Work out the finished part from the listing and answer in its coordinate system (mm). Face numbers are marked on the shaded views. A direction names the side the tool comes from. Round coordinates to 2 decimals unless told otherwise and drop trailing zeros. Loops run counter-clockwise (first coordinate to the right, second up) from the corner with the lowest first, then second, coordinate; pieces in that order, holes last. Notation, with made-up numbers: (31, -4) - (48, -4) arc R18 cw to (48, 19) - close; hole circle Ø10 at (-20.75, 17.25). An arc over 180 degrees is marked (long way). Return JSON: item names as keys, results as strings.
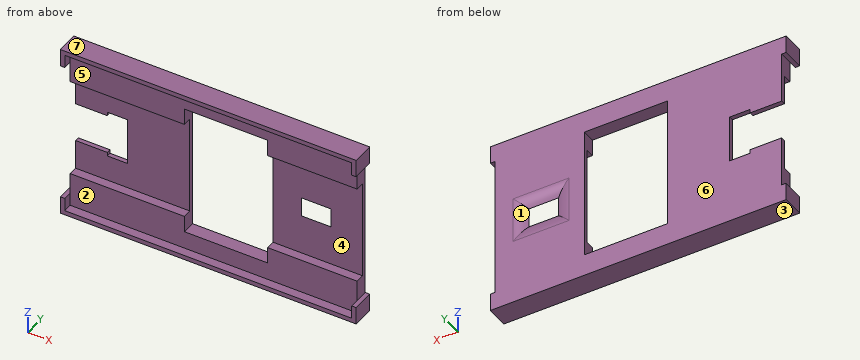
from build123d import *

# Parameters (mm, degrees)
BOSS_EXTRUDE1_DEPTH     = 3
SKETCH2_W               = 6.7
SKETCH2_H               = 4.4
SKETCH2_W_2             = 18.84
SKETCH2_H_2             = 30
CUT_EXTRUDE1_DEPTH      = 77.380625816
CUT_EXTRUDE2_DEPTH      = 61.059054272
CUT_EXTRUDE2_DEPTH_BACK = 61.059054272
SKETCH5_W               = 22.5
SKETCH5_H               = 2
FILLET3_R               = 5
BOSS_EXTRUDE2_DEPTH     = 5


with BuildPart() as part:
    # Sketch1 → Boss-Extrude1 (new body)
    with BuildSketch(Plane(origin=(0, 0, 0), x_dir=(1, 0, 0), z_dir=(0, 1, 0))):
        Polygon((65, -38), (65, -40), (63, -40), (2, -40), (0, -40), (0, -38), (0, -2), (0, 0), (2, 0), (63, 0), (65, 0), (65, -2), align=None)
    extrude(amount=BOSS_EXTRUDE1_DEPTH)

    # Sketch2 → Cut-Extrude1 (cut, through all)
    with BuildSketch(Plane(origin=(0, 3, 0), x_dir=(1, 0, 0), z_dir=(0, 1, 0))):
        with Locations((54.5, -20)):
            Rectangle(SKETCH2_W, SKETCH2_H)
        Polygon((11.78, -25.35), (7.19, -25.35), (7.19, -24.5), (-0.16, -24.5), (-0.16, -15.5), (7.19, -15.5), (7.19, -14.65), (11.78, -14.65), align=None)
        with Locations((35.28, -20)):
            Rectangle(SKETCH2_W_2, SKETCH2_H_2)
    extrude(amount=-CUT_EXTRUDE1_DEPTH, mode=Mode.SUBTRACT)

    # Sketch5 → Cut-Extrude2 (cut, two sides: drawn at the far end of the back side and taken through both)
    with BuildSketch(Plane.ZY.offset(-44.7).offset(-CUT_EXTRUDE2_DEPTH_BACK)):
        with Locations((20, 1)):
            Rectangle(SKETCH5_W, SKETCH5_H)
    extrude(amount=CUT_EXTRUDE2_DEPTH + CUT_EXTRUDE2_DEPTH_BACK, mode=Mode.SUBTRACT)

    # Fillet3
    # the kernel refuses this fillet: 5 mm, written as the material it takes off along each edge
    with BuildSketch(Plane(origin=(57.85, 3, 22.2), x_dir=(0, 0, 1), z_dir=(-1, 0, 0)), Plane(origin=(51.15, 3, 17.8), x_dir=(0, 0, -1), z_dir=(1, 0, 0))) as fillet3_piece_1:
        with BuildLine():
            CenterArc((3, -5), FILLET3_R, 90, 36.869897646)
            Line((0, -1), (-0.06, -0.92))
            ThreePointArc((-0.06, -0.92), (-0.1, -0.5), (-0.1, 0))
            Line((-0.1, 0), (0, 0.1))
            Line((0, 0.1), (3, 0.1))
            Line((3, 0.1), (3, 0))
        make_face()
    extrude(amount=6.7, mode=Mode.SUBTRACT)
    with BuildSketch(Plane(origin=(57.85, 3, 17.8), x_dir=(1, 0, 0), z_dir=(0, 0, 1)), Plane(origin=(51.15, 3, 22.2), x_dir=(-1, 0, 0), z_dir=(0, 0, -1))) as fillet3_piece_2:
        with BuildLine():
            CenterArc((3, -5), FILLET3_R, 90, 36.869897646)
            Line((0, -1), (-0.06, -0.92))
            ThreePointArc((-0.06, -0.92), (-0.1, -0.5), (-0.1, 0))
            Line((-0.1, 0), (0, 0.1))
            Line((0, 0.1), (3, 0.1))
            Line((3, 0.1), (3, 0))
        make_face()
    extrude(amount=4.4, mode=Mode.SUBTRACT)
    with BuildSketch(Plane(origin=(57.85, 3, 17.8), x_dir=(1, 0, 0), z_dir=(0, 0, 1))) as fillet3_piece_3a_section:
        with BuildLine():
            CenterArc((3, -5), FILLET3_R, 90, 36.869897646)
            Line((0, -1), (-0.06, -0.92))
            ThreePointArc((-0.06, -0.92), (-0.1, -0.5), (-0.1, 0))
            Line((-0.1, 0), (0, 0.1))
            Line((0, 0.1), (3, 0.1))
            Line((3, 0.1), (3, 0))
        make_face()
    fillet3_piece_3a = extrude(amount=11.9, mode=Mode.PRIVATE)
    fillet3_piece_3a = split(fillet3_piece_3a, bisect_by=Plane(origin=(58.699672813, 2.773811602, 22.2), z_dir=(0, 0, 1)), keep=Keep.TOP, mode=Mode.PRIVATE)
    with BuildSketch(Plane(origin=(65.35, 3, 22.2), x_dir=(0, 0, 1), z_dir=(-1, 0, 0))) as fillet3_piece_3b_section:
        with BuildLine():
            CenterArc((3, -5), FILLET3_R, 90, 36.869897646)
            Line((0, -1), (-0.06, -0.92))
            ThreePointArc((-0.06, -0.92), (-0.1, -0.5), (-0.1, 0))
            Line((-0.1, 0), (0, 0.1))
            Line((0, 0.1), (3, 0.1))
            Line((3, 0.1), (3, 0))
        make_face()
    fillet3_piece_3b = extrude(amount=14.2, mode=Mode.PRIVATE)
    fillet3_piece_3b = split(fillet3_piece_3b, bisect_by=Plane(origin=(57.85, 2.773811602, 23.049672813), z_dir=(1, 0, 0)), keep=Keep.TOP, mode=Mode.PRIVATE)
    fillet3_piece_3 = fillet3_piece_3a & fillet3_piece_3b
    add(fillet3_piece_3, mode=Mode.SUBTRACT)
    with BuildSketch(Plane(origin=(57.85, 3, 22.2), x_dir=(0, 0, 1), z_dir=(-1, 0, 0))) as fillet3_piece_4a_section:
        with BuildLine():
            CenterArc((3, -5), FILLET3_R, 90, 36.869897646)
            Line((0, -1), (-0.06, -0.92))
            ThreePointArc((-0.06, -0.92), (-0.1, -0.5), (-0.1, 0))
            Line((-0.1, 0), (0, 0.1))
            Line((0, 0.1), (3, 0.1))
            Line((3, 0.1), (3, 0))
        make_face()
    fillet3_piece_4a = extrude(amount=14.2, mode=Mode.PRIVATE)
    fillet3_piece_4a = split(fillet3_piece_4a, bisect_by=Plane(origin=(51.15, 2.773811602, 23.049672813), z_dir=(-1, 0, 0)), keep=Keep.TOP, mode=Mode.PRIVATE)
    with BuildSketch(Plane(origin=(51.15, 3, 29.7), x_dir=(-1, 0, 0), z_dir=(0, 0, -1))) as fillet3_piece_4b_section:
        with BuildLine():
            CenterArc((3, -5), FILLET3_R, 90, 36.869897646)
            Line((0, -1), (-0.06, -0.92))
            ThreePointArc((-0.06, -0.92), (-0.1, -0.5), (-0.1, 0))
            Line((-0.1, 0), (0, 0.1))
            Line((0, 0.1), (3, 0.1))
            Line((3, 0.1), (3, 0))
        make_face()
    fillet3_piece_4b = extrude(amount=11.9, mode=Mode.PRIVATE)
    fillet3_piece_4b = split(fillet3_piece_4b, bisect_by=Plane(origin=(50.300327187, 2.773811602, 22.2), z_dir=(0, 0, 1)), keep=Keep.TOP, mode=Mode.PRIVATE)
    fillet3_piece_4 = fillet3_piece_4a & fillet3_piece_4b
    add(fillet3_piece_4, mode=Mode.SUBTRACT)
    with BuildSketch(Plane(origin=(51.15, 3, 17.8), x_dir=(0, 0, -1), z_dir=(1, 0, 0))) as fillet3_piece_5a_section:
        with BuildLine():
            CenterArc((3, -5), FILLET3_R, 90, 36.869897646)
            Line((0, -1), (-0.06, -0.92))
            ThreePointArc((-0.06, -0.92), (-0.1, -0.5), (-0.1, 0))
            Line((-0.1, 0), (0, 0.1))
            Line((0, 0.1), (3, 0.1))
            Line((3, 0.1), (3, 0))
        make_face()
    fillet3_piece_5a = extrude(amount=14.2, mode=Mode.PRIVATE)
    fillet3_piece_5a = split(fillet3_piece_5a, bisect_by=Plane(origin=(57.85, 2.773811602, 16.950327187), z_dir=(1, 0, 0)), keep=Keep.TOP, mode=Mode.PRIVATE)
    with BuildSketch(Plane(origin=(57.85, 3, 10.3), x_dir=(1, 0, 0), z_dir=(0, 0, 1))) as fillet3_piece_5b_section:
        with BuildLine():
            CenterArc((3, -5), FILLET3_R, 90, 36.869897646)
            Line((0, -1), (-0.06, -0.92))
            ThreePointArc((-0.06, -0.92), (-0.1, -0.5), (-0.1, 0))
            Line((-0.1, 0), (0, 0.1))
            Line((0, 0.1), (3, 0.1))
            Line((3, 0.1), (3, 0))
        make_face()
    fillet3_piece_5b = extrude(amount=11.9, mode=Mode.PRIVATE)
    fillet3_piece_5b = split(fillet3_piece_5b, bisect_by=Plane(origin=(58.699672813, 2.773811602, 17.8), z_dir=(0, 0, -1)), keep=Keep.TOP, mode=Mode.PRIVATE)
    fillet3_piece_5 = fillet3_piece_5a & fillet3_piece_5b
    add(fillet3_piece_5, mode=Mode.SUBTRACT)
    with BuildSketch(Plane(origin=(43.65, 3, 17.8), x_dir=(0, 0, -1), z_dir=(1, 0, 0))) as fillet3_piece_6a_section:
        with BuildLine():
            CenterArc((3, -5), FILLET3_R, 90, 36.869897646)
            Line((0, -1), (-0.06, -0.92))
            ThreePointArc((-0.06, -0.92), (-0.1, -0.5), (-0.1, 0))
            Line((-0.1, 0), (0, 0.1))
            Line((0, 0.1), (3, 0.1))
            Line((3, 0.1), (3, 0))
        make_face()
    fillet3_piece_6a = extrude(amount=14.2, mode=Mode.PRIVATE)
    fillet3_piece_6a = split(fillet3_piece_6a, bisect_by=Plane(origin=(51.15, 2.773811602, 16.950327187), z_dir=(-1, 0, 0)), keep=Keep.TOP, mode=Mode.PRIVATE)
    with BuildSketch(Plane(origin=(51.15, 3, 22.2), x_dir=(-1, 0, 0), z_dir=(0, 0, -1))) as fillet3_piece_6b_section:
        with BuildLine():
            CenterArc((3, -5), FILLET3_R, 90, 36.869897646)
            Line((0, -1), (-0.06, -0.92))
            ThreePointArc((-0.06, -0.92), (-0.1, -0.5), (-0.1, 0))
            Line((-0.1, 0), (0, 0.1))
            Line((0, 0.1), (3, 0.1))
            Line((3, 0.1), (3, 0))
        make_face()
    fillet3_piece_6b = extrude(amount=11.9, mode=Mode.PRIVATE)
    fillet3_piece_6b = split(fillet3_piece_6b, bisect_by=Plane(origin=(50.300327187, 2.773811602, 17.8), z_dir=(0, 0, -1)), keep=Keep.TOP, mode=Mode.PRIVATE)
    fillet3_piece_6 = fillet3_piece_6a & fillet3_piece_6b
    add(fillet3_piece_6, mode=Mode.SUBTRACT)

    # Sketch8 → Boss-Extrude2 (add)
    with BuildSketch(Plane(origin=(0, 3, 0), x_dir=(1, 0, 0), z_dir=(0, 1, 0))):
        Polygon((-1, -40), (66, -40), (66, -39), (66, -36), (65, -36), (65, -39), (0, -39), (0, -36), (-1, -36), (-1, -39), align=None)
        Polygon((-1, 0), (66, 0), (66, -1), (66, -4), (65, -4), (65, -1), (0, -1), (0, -4), (-1, -4), (-1, -1), align=None)
    extrude(amount=-BOSS_EXTRUDE2_DEPTH)


solid = part.part
1) Flat-ended cylindrical pins translate along their axes: pin 1 (0.7 mm diameter, centred on y = 2.5, z = 24.5, fed in from +X); pin 2 (10 mm diameter, centred on x = 50.5, z = 14.5, fed in from -Y); pin 3 (0.5 mm diameter, centred on y = 2.5, z = 21.5, fed in from -X). Find the tip coordinate at first contact, or state that the pin passes through.
Verdict:
{"pin 1": "stops at x = 65", "pin 2": "stops at y = 2", "pin 3": "stops at x = 11.78"}
2) Find the intervals of material crossed by L1, parallel to Z at x = 17, y = -1.55; L2, parallel to Z at x = 40.5, y = 1.4; L3, parallel to X at y = -1.25, z = 36.5, in increasing order.
Verdict:
{"L1": "z = 0 to 1, 39 to 40", "L2": "z = 0 to 5, 35 to 40", "L3": "x = -1 to 0, 65 to 66"}
3) Section A-A (x = 9.5) is taken. Give the vertices of the cut face in (y, z), and give its area (3 significant figures).
Verdict:
{"outline": "(-2, 0) - (3, 0) - (3, 14.65) - (2, 14.65) - (2, 8.75) - (0, 8.75) - (0, 1) - (-2, 1) - close; (-2, 39) - (0, 39) - (0, 31.25) - (2, 31.25) - (2, 25.35) - (3, 25.35) - (3, 40) - (-2, 40) - close", "area": "68.3 mm2"}
4) Section D-D (x = 39) is taken. Give the vertices of the cut face in (y, z), and give its area (3 significant figures).
Verdict:
{"outline": "(-2, 0) - (3, 0) - (3, 5) - (0, 5) - (0, 1) - (-2, 1) - close; (-2, 39) - (0, 39) - (0, 35) - (3, 35) - (3, 40) - (-2, 40) - close", "area": "34.0 mm2"}
5) Determine the mould class of the marked faces 5, 6 and 7 for opening direction Z: pulls with the +Z half, pulls with the -Z half, needs draft (parallel to the pull), parting line crosses it, or undercut.
Verdict:
{"face 5": "undercut", "face 6": "needs draft", "face 7": "pulls with the +Z half"}
6) Section B-B (z = 32.5) is taken. Give the vertices of the cut face in (x, y).
Verdict:
{"outline": "(0, 0) - (25.86, 0) - (25.86, 3) - (0, 3) - close; (44.7, 0) - (65, 0) - (65, 3) - (44.7, 3) - close"}
7) Section C-C (y = -1.15) is taken. Give the vertices of the cut face in (x, z), and give its area (3 significant figures).
Verdict:
{"outline": "(-1, 0) - (66, 0) - (66, 4) - (65, 4) - (65, 1) - (0, 1) - (0, 4) - (-1, 4) - close; (-1, 36) - (0, 36) - (0, 39) - (65, 39) - (65, 36) - (66, 36) - (66, 40) - (-1, 40) - close", "area": "146 mm2"}
8) A tool of negligible diameter and unlimited length cuts with its end or side. For the marked faces 1, 2, 3 and 4, from which of +Z, -Z, +X, -X, +Y, -Y can it reach the whole face along a straight path? Write none if from no direction.
Verdict:
{"face 1": "+Y", "face 2": "-Y", "face 3": "-Z, +X, -X, +Y, -Y", "face 4": "+X, -X, -Y"}
